The drawing under review shows one solid part. Ordinate dimensions are in mm from its lowest x, y, z. A direction names the side the tool comes from. Coordinates: 2 decimals unless noted, no trailing zeros. Write each loop counter-clockwise with the first axis right and the second up, starting at its lowest first coordinate (ties: lowest second). Pieces come first, ordered by that corner, then holes. Notation, with made-up numbers: M -20,-29 L 26,-29 A20 ccw 26,-2 Z; hole C -11.5,11.5 d10. An arc over 180 degrees is marked long. Write item = value, one per line.
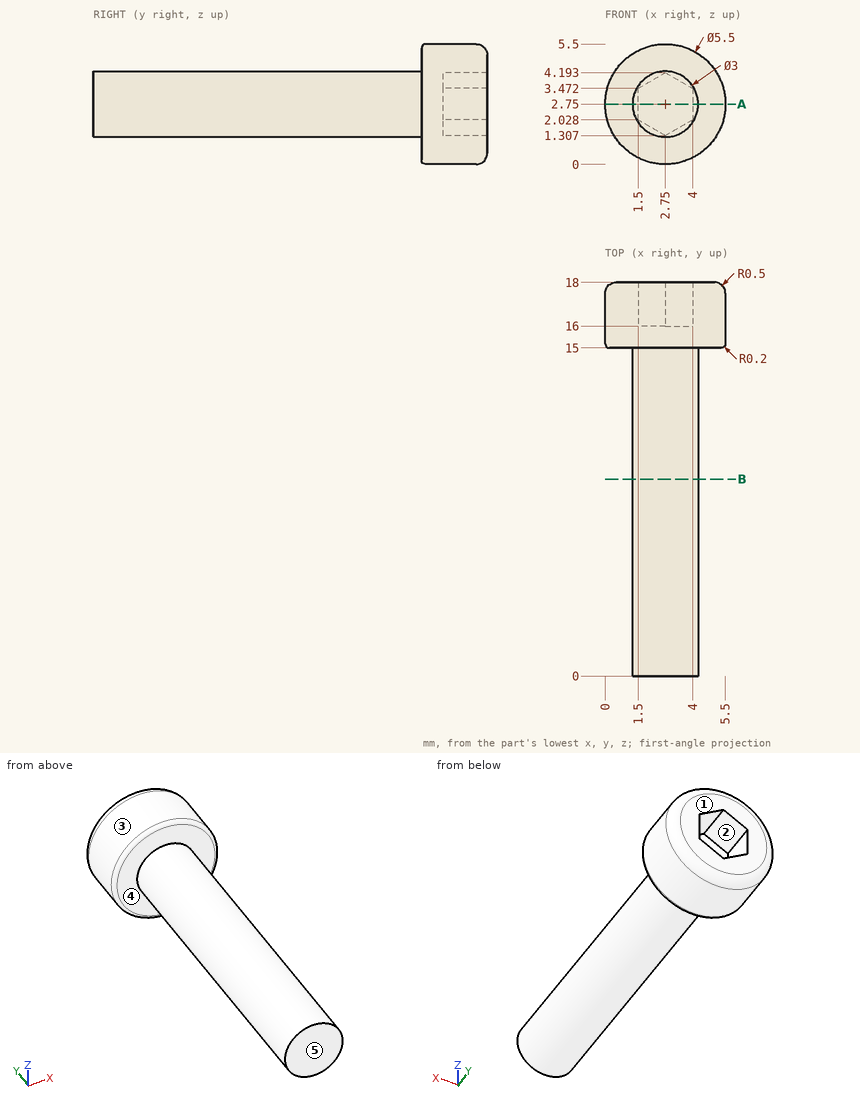
Q1. Consider section A-A, the plane z = 2.75. State the section outline as (x, y) points.
Check result:
outline = M 0,15.2 A0.2 ccw 0.2,15 L 1.25,15 L 1.25,0 L 4.25,0 L 4.25,15 L 5.3,15 A0.2 ccw 5.5,15.2 L 5.5,17.5 A0.5 ccw 5,18 L 4,18 L 4,16 L 1.5,16 L 1.5,18 L 0.5,18 A0.5 ccw 0,17.5 Z
Q2. Wall thickness on line 1 (Y direction, x = 2.4, z = 3.3); line 2 (Z direction, x = 1.75, y = 17) (1 decimal); line 3 (Y direction, x = 2.3, z = 4.6): over which ranges is each line inside the solid? List them lowest first.
Check result:
line_1 = 0 to 16
line_2 = 0.2 to 1.9, 3.6 to 5.3
line_3 = 15 to 18
Q3. For P1, Ø1.5, axis at x = 1, y = 7, coming from the +Z side; P2, Ø2, axis at x = 5, z = 1.5, coming from the -Y side; P3, Ø0.8, axis at x = 2.5, z = 2.5, coming from the +Y side, all flat-tipped, find the tip position at first contact; note any pin that passes through.
Check result:
P1 = 3.87
P2 = 15
P3 = 16
Q4. Machinability: for the marked faces 4 and 5, which of the approach directions +Z, -Z, +X, -X, +Y, -Y give a long, thin tool a straight path to every point of the face, cutting with its end or side? Answer none if there is none.
Check result:
face_4 = -Y
face_5 = +Z, -Z, +X, -X, -Y
Q5. Consider section B-B, the plane y = 9. State the section outline as (x, z) points.
Check result:
outline = C 2.75,2.75 d3
Q6. The part is to be moulded in two halves that separate along Z. For the marked faces 1, 2 and 3, say which applies: +Z half, -Z half, draft (parallel to the pull), parting line (faces both ways), or undercut.
Check result:
face_1 = draft
face_2 = undercut
face_3 = parting line
